```python
from build123d import *

# Parameters (mm, degrees)
F0_W         = 152.4
F0_H         = 50.8
F0_W_2       = 33.4925577044
F0_H_2       = 31.1666876078
F1_DEPTH     = 63.5
F3_DEPTH     = 26.67
F2_W         = 163.8920905882
F2_H         = 5.08
F4_DEPTH     = 27.94
F2_W_2       = 10.0997969608
F2_H_2       = 12.7
F5_DEPTH     = 29.21
F6_T4_DEPTH  = 152.4
F6_T9_DEPTH  = 152.4
F6_T14_DEPTH = 38.8282991577
F7_T4_DEPTH  = 82.0082991577
F8_SIZE      = 5.08
F9_SIZE      = 5.08
F10_R        = 4.2050090424
F11_DEPTH    = 33.528
F12_W        = 147.32
F12_H        = 11.7464326172
F13_DEPTH    = 26.67
F14_R        = 8.4361197875
F15_DEPTH    = 82.296


# Not quite as in the source:
# - a fillet or chamfer that OpenCascade refuses, or shapes differently, is made with other operations: its cross-section is extruded or revolved along the edge and cut away or added


with BuildPart() as f1:
    # F0 (on Top) → F1 (new body)
    with BuildSketch(Plane.XY):
        Rectangle(F0_W, F0_H)
        with Locations((42.3862338066, 0)):
            Rectangle(F0_W_2, F0_H_2, mode=Mode.SUBTRACT)
    extrude(amount=F1_DEPTH)

    # F2 (on Front) → F3 (join, symmetric)
    with BuildSketch(Plane.XZ):
        Polygon((77.0109159804, 0), (-77.9290840196, 0), (-77.9290840196, -12.7), (4.4760434559, -12.7), (65.76342, -12.7), (77.0109159804, -12.7), align=None)
    extrude(amount=F3_DEPTH, both=True)

    # F2 (on Front) → F4 (join, symmetric)
    with BuildSketch(Plane.XZ):
        with Locations((5.1646676471, 65.5489305882)):
            Rectangle(F2_W, F2_H)
    extrude(amount=F4_DEPTH, both=True)

    # F2 (on Front) → F5 (join, symmetric)
    with BuildSketch(Plane.XZ):
        with Locations((82.0608144608, -6.35)):
            Rectangle(F2_W_2, F2_H_2)
    extrude(amount=F5_DEPTH, both=True)

    # F6: chamfer of 5.08 on 3 edges, made by hand


with BuildPart() as f6_tool2:
    # F6_s3 → F6_t4 (new body)
    with BuildSketch(Plane.YZ.offset(76.2)):
        Polygon((-25.4, 57.9289305882), (-30.48, 63.0089305882), (-25.4, 63.0089305882), align=None)
    extrude(amount=-F6_T4_DEPTH)

    split(bisect_by=Plane.XZ.offset(27.94), keep=Keep.BOTTOM)


with BuildPart() as f1_1:
    add(f1.part)

    # F6_t1: union F6_tool2
    add(f6_tool2.part)


with BuildPart() as f6_tool7:
    # F6_s8 → F6_t9 (new body)
    with BuildSketch(Plane.YZ.offset(-76.2)):
        Polygon((25.4, 57.9289305882), (30.48, 63.0089305882), (25.4, 63.0089305882), align=None)
    extrude(amount=F6_T9_DEPTH)

    split(bisect_by=Plane.XZ.offset(-27.94), keep=Keep.TOP)


with BuildPart() as f1_2:
    add(f1_1.part)

    # F6_t6: union F6_tool7
    add(f6_tool7.part)


with BuildPart() as f6_tool12:
    # F6_s13 → F6_t14 (new body)
    with BuildSketch(Plane.XY.offset(13.0641495789)):
        Polygon((82.0909159804, -29.21), (77.0109159804, -24.13), (77.0109159804, -29.21), align=None)
    extrude(amount=-F6_T14_DEPTH)

    split(bisect_by=Plane.XZ.offset(26.67), keep=Keep.TOP)


with BuildPart() as f1_3:
    add(f1_2.part)

    # F6_t11: cut F6_tool12
    add(f6_tool12.part, mode=Mode.SUBTRACT)

    # F7: chamfer of 5.08 on 1 edges, made by hand


with BuildPart() as f7_tool2:
    # F7_s3 → F7_t4 (new body)
    with BuildSketch(Plane.XZ.offset(-41.0041495789)):
        Polygon((-71.7013776471, 63.0089305882), (-76.7813776471, 68.0889305882), (-76.7813776471, 63.0089305882), align=None)
    extrude(amount=F7_T4_DEPTH)

    split(bisect_by=Plane.YZ.offset(-76.2), keep=Keep.BOTTOM)


with BuildPart() as f1_4:
    add(f1_3.part)

    # F7_t1: cut F7_tool2
    add(f7_tool2.part, mode=Mode.SUBTRACT)

    # F8
    f8_edges = [f1_4.edges().sort_by_distance(p)[0] for p in [
        (76.2, 0, 63.008931),
    ]]
    chamfer(f8_edges, length=F8_SIZE)

    # F9
    f9_edges = [f1_4.edges().sort_by_distance(p)[0] for p in [
        (81.28, 0, 63.008931),
    ]]
    chamfer(f9_edges, length=F9_SIZE)

    # F10 (on Front) → F11 (join)
    with BuildSketch(Plane.XZ):
        with Locations((-65.0145885289, 45.2289305882)):
            Circle(F10_R)
        with Locations((-39.6145885289, 45.2289305882)):
            Circle(F10_R)
        with Locations((-14.2145885289, 45.2289305882)):
            Circle(F10_R)
        with Locations((11.1854114711, 45.2289305882)):
            Circle(F10_R)
        with Locations((36.5854114711, 45.2289305882)):
            Circle(F10_R)
        with Locations((61.9854114711, 45.2289305882)):
            Circle(F10_R)
    extrude(amount=F11_DEPTH)

    # F12 (on Front) → F13 (join)
    with BuildSketch(Plane.XZ):
        with Locations((0, 44.957723322)):
            Rectangle(F12_W, F12_H)
    extrude(amount=F13_DEPTH)

    # F14 (on Right) → F15 (join)
    with BuildSketch(Plane.YZ):
        Circle(F14_R)
    extrude(amount=F15_DEPTH)


solid = f1_4.part
```
Read the model definition and answer for the solid it produces. Units are mm, in the model's axes. A direction names the side the tool comes from. Give positions to 0.01 mm unless a question says otherwise; leave off trailing zeros. Write each loop counter-clockwise with the first axis right and the second up, starting at its lowest first coordinate (ties: lowest second). Pieces come first, ordered by that corner, then holes. Notation, with made-up numbers: M 2.25,11.25 L 61.25,11.25 A20 cw 61.25,20.25 Z; hole C -32.5,39.25 d2. An arc over 180 degrees is marked long. Put each result on its own line as item: value. Start each with the question number.
1. Consider line 1 along Z through (x, y) = (27, -12); line 2 along X through (y, z) = (-3.5, 16); line 3 along X through (y, z) = (16.5, 12). Determine where each line is inside the solid, lowest interval first.
2. Which of the six approach directions +Z, -Z, +X, -X, +Y, -Y give full straight-line access (tool end or side, diameter ignored) to faces 3 (the flat face through (-1, -26.67, 45)), 4 (the flat face through (4, -27.94, 64)), 5 (the flat face through (82.085, 0.391, 61.238))?
3. Each of these flat-tipped pins is pushed along its axis until it touches: pin 1 Ø9.5 at (y, z) = (-1, 22) entering from -X; pin 2 Ø4 at (x, z) = (-22.5, 64) entering from -Y; pin 3 Ø3.5 at (x, z) = (46.5, 46.5) entering from +Y. Where does it stop, or does it pass through?
4. For a pull along Z with two mould halves and no side action, classify faces 1 (the flat face through (11, -33.528, 45)), 2 (the flat face through (42, 0, 45)) as released by +Z, released by -Z, zero draft, split by the parting line, or undercut.
5. The part is cut by section C-C, the plane x = 10.5. Give the vertices of the cut face in (y, z).
6. The part is cut by section B-B, the plane z = 36. Give the vertices of the cut face in (x, y).
7. The part is cut by section A-A, the plane y = 13.5. Give the vertices of the cut face in (x, z), and give its area (3 significant figures).
Final values:
1. line 1: z = -12.7 to 0, 39.08 to 50.83, 63.01 to 68.09
1. line 2: x = -76.2 to 25.64, 59.13 to 76.2
1. line 3: x = -76.2 to 76.2
2. face 3: -Y
2. face 4: +Z, +X, -X, -Y
2. face 5: +X, +Y, -Y
3. pin 1: stops at x = -76.2
3. pin 2: stops at y = -27.94
3. pin 3: stops at y = 25.4
4. face 1: zero draft
4. face 2: undercut
5. outline: M -33.53,41.08 L -26.67,41.08 L -26.67,39.08 L -25.4,39.08 L -25.4,0 L -26.67,0 L -26.67,-12.7 L 26.67,-12.7 L 26.67,0 L 25.4,0 L 25.4,57.93 L 27.94,60.47 L 27.94,68.09 L -27.94,68.09 L -27.94,60.47 L -25.4,57.93 L -25.4,50.83 L -26.67,50.83 L -26.67,49.38 L -33.53,49.38 Z
6. outline: M -76.2,-25.4 L 76.2,-25.4 L 76.2,25.4 L -76.2,25.4 Z; hole M 25.64,-15.58 L 59.13,-15.58 L 59.13,15.58 L 25.64,15.58 Z
7. outline: M -77.93,-12.7 L 87.11,-12.7 L 87.11,0 L 76.2,0 L 76.2,57.93 L 77.69,59.42 L 86.36,63.01 L 87.11,63.01 L 87.11,68.09 L -76.78,68.09 L -76.2,67.51 L -76.2,0 L -77.93,0 Z; hole M 25.64,0 L 59.13,0 L 59.13,63.01 L 25.64,63.01 Z
7. area: 10,400 mm²
